CAD build for the part. Positions are in the model's coordinates, mm. A direction names the side the tool comes from. Round coordinates to 2 decimals unless told otherwise and drop trailing zeros. Order: outer loops, then holes, each group sorted by start corner. A loop starts at its lowest first (then second) coordinate and runs counter-clockwise, first axis right, second up. Notation, with made-up numbers: M -22.5,60.5 L -18.5,60.5 A18 cw -18.5,73.5 Z; hole C -4.75,-37 d2. An arc over 180 degrees is marked long. Answer as a JSON object with one key per item and string values.
Autodesk Inventor part; units mm, degrees
ref_plane "YZ Plane" through (0, 0, 0) normal (1, 0, 0) x (0, 1, 0)
ref_plane "XZ Plane" through (0, 0, 0) normal (0, 1, 0) x (-1, 0, 0)
ref_plane "XY Plane" through (0, 0, 0) normal (0, 0, 1) x (1, 0, 0)
sketch "スケッチ1" plane through (0, 0, 0) normal (0, 0, 1) x (1, 0, 0)
  line L0 (-10, 20) -> (10, 20) construction
  line L1 (10, 20) -> (10, -20) construction
  line L2 (10, -20) -> (-10, -20) construction
  line L3 (-10, -20) -> (-10, 20) construction
  line L4 (-10, 20) -> (10, -20) construction
  line L5 (10, 20) -> (-10, -20) construction
  circle A0 centre (-7.25, 17.25) radius 1.75
  line L6 (0, 20) -> (0, -20) construction
  circle A1 centre (7.25, 17.25) radius 1.75
  line L7 (9, -19) -> (-9, -19)
  line L8 (-9, -19) -> (-9, 14.8133)
  line L9 (-9, 19) -> (-4.8133, 19) construction
  line L10 (9, 19) -> (9, 14.8133) construction
  line L11 (9, -19) -> (-9, 19) construction
  line L12 (-9, -19) -> (9, 19) construction
  arc A2 (-9, 14.8133) -> (-4.8133, 19) centre (-7.25, 17.25) ccw
  line L13 (-4.8133, 19) -> (4.8133, 19)
  line L14 (-9, 14.8133) -> (-9, 19) construction
  arc A3 (4.8133, 19) -> (9, 14.8133) centre (7.25, 17.25) ccw
  line L15 (4.8133, 19) -> (9, 19) construction
  line L16 (9, 14.8133) -> (9, -19)
  line L17 (-11, 21) -> (11, 21)
  line L18 (11, 21) -> (11, -21)
  line L19 (11, -21) -> (-11, -21)
  line L20 (-11, -21) -> (-11, 21)
  line L21 (-11, 21) -> (11, -21) construction
  line L22 (11, 21) -> (-11, -21) construction
  line L23 (10.25, -20.25) -> (-10.25, -20.25)
  line L24 (-10.25, -20.25) -> (-10.25, 20.25)
  line L25 (-10.25, 20.25) -> (10.25, 20.25)
  line L26 (10.25, 20.25) -> (10.25, -20.25)
  line L27 (10.25, -20.25) -> (-10.25, 20.25) construction
  line L28 (-10.25, -20.25) -> (10.25, 20.25) construction
  point P0 (0, 0)
  point P1 (0, 0)
  dimension "d0" = 20
  dimension "d1" = 40
  dimension "d2" = 3.5
  dimension "d3" = 2.75
  dimension "d4" = 2.75
  dimension "d5" = 1
  dimension "d6" = 1
  dimension "d7" = 3
  dimension "d13" = 1
  dimension "d14" = 1
  dimension "d15" = 0.25
  dimension "d16" = 0.25
extrude "押し出し1" add sketch "スケッチ1" along normal blind 6.6 contours L17 L18 L19 L20
extrude "押し出し2" add sketch "スケッチ1" along normal blind 1 contours L7 L8 A2 L13 A3 L16 | L23 L24 L25 L26
extrude "押し出し3" add sketch "スケッチ1" along normal blind 5 contours L17 L18 L19 L20 | L23 L24 L25 L26
fillet "フィレット1" radius 2 6 edges at (-9, 14.8133, 3) (-4.8133, 19, 3) (4.8133, 19, 3) (9, 14.8133, 3) (-9, -19, 3) (9, -19, 3)
equation "\"d4\" = d3"
equation "\"d6\" = d5"
equation "\"d14\" = d5"
properties part number "_3D プリント"
Item 1: Saw through at D-D on x = -8.5. List the corners of the cut face in (y, z), and give its area (3 significant figures).
Worked answers:
{"outline": "M -21,0 L 16.03,0 L 16.03,5 L 13.58,5 L 13.58,1 L -18.32,1 L -18.32,5 L -20.25,5 L -20.25,6.6 L -21,6.6 Z; M 18.47,0 L 21,0 L 21,6.6 L 20.25,6.6 L 20.25,5 L 18.47,5 Z", "area": "72.5 mm2"}
Item 2: 3-axis set-ups, long thin cutter, end or side, ignore diameter. For faces 5 (the flat face through (0, -21, 3)), 6 (the flat face through (0, 0, 1)): which of +Z, -Z, +X, -X, +Y, -Y reach the whole face in a straight line?
Worked answers:
{"face 5": "+Z, -Z, +X, -X, -Y", "face 6": "+Z"}
Item 3: Saw through at C-C on z = 6. List the corners of the cut face in (x, y), and give its area (4 significant figures).
Worked answers:
{"outline": "M -11,-21 L 11,-21 L 11,21 L -11,21 Z; hole M -10.25,-20.25 L 10.25,-20.25 L 10.25,20.25 L -10.25,20.25 Z", "area": "93.75 mm2"}
Item 4: Two-plate mould, pull along Y, no slides. Class faces 1 (the flat face through (-11, 0, 3)), 2 (the cylindrical face through (8.4, -18.43, 3.03)), 3 (the flat face through (0, 20.25, 6)), 4 (the flat face through (0, 21, 3)): released by +Y, released by -Y, zero draft, split by the parting line, or undercut.
Worked answers:
{"face 1": "zero draft", "face 2": "undercut", "face 3": "undercut", "face 4": "released by +Y"}
Item 5: Drop flat-ended pins along their axis: pin 1 Ø2 at (x, y) = (2, 6.5) entering from +Z; pin 2 Ø8 at (x, y) = (5.5, -6) entering from +Z; pin 3 Ø3 at (x, y) = (-7.25, 17.25) entering from -Z; pin 4 Ø5.5 at (x, y) = (7.25, 17.25) entering from -Z. Give the stop position or say it passes through.
Worked answers:
{"pin 1": "stops at z = 1", "pin 2": "stops at z = 5", "pin 3": "passes through", "pin 4": "stops at z = 0"}
Item 6: Wall check: line 1 along Y through (x, z) = (-4.25, 6); line 2 along X through (y, z) = (0, 4); line 3 along Y through (x, z) = (7.25, 1.65). Give the ranges that are in metal, low to high. Write a range as [from, to].
Worked answers:
{"line 1": "y = [-21, -20.25], [20.25, 21]", "line 2": "x = [-11, -9], [9, 11]", "line 3": "y = [-21, -18.98], [14.24, 15.5], [19, 21]"}
Item 7: Saw through at A-A on z = 3.25. List the corners of the cut face in (x, y), and give its area (3 significant figures).
Worked answers:
{"outline": "M -11,-21 L 11,-21 L 11,21 L -11,21 Z; hole M -9,-17 A2 ccw -7,-19 L 7,-19 A2 ccw 9,-17 L 9,12.26 A2 ccw 7.1,14.25 A3 cw 4.25,17.1 A2 ccw 2.26,19 L -2.26,19 A2 ccw -4.25,17.1 A3 cw -7.1,14.25 A2 ccw -9,12.26 Z; hole C -7.25,17.25 d3.5; hole C 7.25,17.25 d3.5", "area": "267 mm2"}
Item 8: Saw through at B-B on y = -12.5. List the corners of the cut face in (x, z), and give its area (3 significant figures).
Worked answers:
{"outline": "M -11,0 L 11,0 L 11,6.6 L 10.25,6.6 L 10.25,5 L 9,5 L 9,1 L -9,1 L -9,5 L -10.25,5 L -10.25,6.6 L -11,6.6 Z", "area": "40.4 mm2"}
